from build123d import *

# Parameters (mm, degrees)
SKETCH1_W           = 200
SKETCH1_H           = 150
SKETCH1_W_2         = 192
SKETCH1_H_2         = 142
BOSS_EXTRUDE2_DEPTH = 4
SKETCH2_W           = 200
SKETCH2_H           = 150
SKETCH2_W_2         = 192
SKETCH2_H_2         = 142
BOSS_EXTRUDE3_DEPTH = 80
CUT_EXTRUDE1_DEPTH  = 150


with BuildPart() as part:
    # Sketch1 → Boss-Extrude2 (new body)
    # profile 1 of 3: a face of its own
    with BuildSketch(Plane(origin=(0, 0, 0), x_dir=(1, 0, 0), z_dir=(0, 1, 0))):
        with Locations((-100, 75)):
            Rectangle(SKETCH1_W, SKETCH1_H)
        with Locations((-100, 75)):
            Rectangle(SKETCH1_W_2, SKETCH1_H_2, mode=Mode.SUBTRACT)
    # profile 2 of 3: a face of its own
    with BuildSketch(Plane(origin=(0, 0, 0), x_dir=(1, 0, 0), z_dir=(0, 1, 0))):
        Polygon((-4, 75), (-196, 75), (-196, 44), (-171, 44), (-171, 64), (-163, 64), (-163, 74), (-159, 74), (-159, 64), (-151, 64), (-151, 44), (-126, 44), (-126, 4), (-4, 4), align=None)
    # profile 3 of 3: a face of its own
    with BuildSketch(Plane(origin=(0, 0, 0), x_dir=(1, 0, 0), z_dir=(0, 1, 0))):
        Polygon((-196, 106), (-196, 75), (-4, 75), (-4, 146), (-126, 146), (-126, 106), (-151, 106), (-151, 86), (-159, 86), (-159, 76), (-163, 76), (-163, 86), (-171, 86), (-171, 106), align=None)
    extrude(amount=BOSS_EXTRUDE2_DEPTH)

    # Sketch2 → Boss-Extrude3 (add)
    with BuildSketch(Plane(origin=(0, 4, 0), x_dir=(1, 0, 0), z_dir=(0, 1, 0))):
        with Locations((-100, 75)):
            Rectangle(SKETCH2_W, SKETCH2_H)
        with Locations((-100, 75)):
            Rectangle(SKETCH2_W_2, SKETCH2_H_2, mode=Mode.SUBTRACT)
    extrude(amount=BOSS_EXTRUDE3_DEPTH)

    # Sketch3 → Cut-Extrude1 (cut)
    with BuildSketch(Plane.XY):
        Polygon((-200, 84), (0, 14), (0, 84), align=None)
    extrude(amount=-CUT_EXTRUDE1_DEPTH, mode=Mode.SUBTRACT)


solid = part.part
The model under review builds one solid part; all positions refer to its coordinate system, in mm. A direction names the side the tool comes from. Give positions to 0.01 mm unless a question says otherwise; leave off trailing zeros. Order: outer loops, then holes, each group sorted by start corner. A loop starts at its lowest first (then second) coordinate and runs counter-clockwise, first axis right, second up. Notation, with made-up numbers: (60.5, 72.5) -> (105.5, 72.5) arc R31 ccw to (105.5, 108.5) -> close; hole circle Ø9 at (69.25, -25.5). An arc over 180 degrees is marked (long way). Write item = value, one per line. Start each with the question number.
(1) Take a section at D-D (x = -23). Write out the cut boundary in (y, z).
(2) For pin 1 Ø3 at (y, z) = (36, -114.5) entering from +X; pin 2 Ø2 at (x, z) = (-95.5, -108.5) entering from +Y, all flat-tipped, find the tip position at first contact; note any pin that passes through.
(3) Draft analysis for pull direction Z (two halves, no side actions). For faces 4 (the flat face through (-184, 2, -44)), 5 (the flat face through (0, 7, -74)), 6 (the flat face through (-124, 32, -150)), state which applies: +Z half, -Z half, draft (parallel to the pull), parting line (faces both ways), or undercut.
(4) Take a section at C-C (y = 77). Write out the cut boundary in (x, z).
(5) Take a section at A-A (x = -168). Write out the cut boundary in (y, z), plus the area to 3 significant figures.
(6) For L1, parallel to X at y = 9.5, z = -98.5; L2, parallel to Z at x = -102, y = 33; L3, parallel to Y at x = -8, z = -64, list the stretches that pass through material, from the lowest coordinate up. Write a range as from..to.
(7) Tool access review of faces 1 (the flat face through (-124, 32, 0)), 2 (the flat face through (-171, 2, -96)), 3 (the flat face through (-123, 32, -146)): name each direction out of +Z, -Z, +X, -X, +Y, -Y from which nothing blocks a thin tool from reaching the whole face with its end or side.
(8) Take a section at B-B (z = -27.5). Write out the cut boundary in (x, y), plus the area to 3 significant figures.
Returned:
q1.outline = (0, -150) -> (22.05, -150) -> (22.05, -146) -> (4, -146) -> (4, -4) -> (22.05, -4) -> (22.05, 0) -> (0, 0) -> close
q2.pin_1 = -196
q2.pin_2 = 4
q3.face_4 = undercut
q3.face_5 = draft
q3.face_6 = -Z half
q4.outline = (-200, -150) -> (-180, -150) -> (-180, -146) -> (-196, -146) -> (-196, -4) -> (-180, -4) -> (-180, 0) -> (-200, 0) -> close
q5.outline = (0, -150) -> (72.8, -150) -> (72.8, -146) -> (0, -146) -> close; (0, -86) -> (4, -86) -> (4, -64) -> (0, -64) -> close; (0, -4) -> (72.8, -4) -> (72.8, 0) -> (0, 0) -> close
q5.area = 670 mm²
q6.L1 = -200..-196, -4..0
q6.L2 = -150..-146, -4..0
q6.L3 = 0..4
q7.face_1 = +Z, +X, -X, +Y, -Y
q7.face_2 = +Y, -Y
q7.face_3 = +Y
q8.outline = (-200, 0) -> (-196, 0) -> (-196, 82.6) -> (-200, 84) -> close; (-126, 0) -> (0, 0) -> (0, 14) -> (-4, 15.4) -> (-4, 4) -> (-126, 4) -> close
q8.area = 880 mm²
